Check sheet for the modelled part. Datum: model origin and axes. Units: mm. Face numbers are marked on the shaded views. A direction names the side the tool comes from. Round coordinates to 2 decimals unless told otherwise and drop trailing zeros. Write each loop counter-clockwise with the first axis right and the second up, starting at its lowest first coordinate (ties: lowest second). Pieces come first, ordered by that corner, then holes.
Item 1: Material ranges on line 1 along Z through (x, y) = (9.5, 5); line 2 along Y through (x, z) = (10, 6); line 3 along Z through (x, y) = (16.2, -19.05), recorded low to high.
Item 2: Section check A-A, the plane y = -0.5. Record the cut outline in (x, z), plus the area to 3 significant figures.
Item 3: Release check for a two-part mould opening along Z. For the marked faces 1, 2 and 3 record: pulls with the +Z half, pulls with the -Z half, needs draft (parallel to the pull), parting line crosses it, or undercut.
Item 4: Section check B-B, the plane x = 16.2. Record the cut outline in (y, z), plus the area to 3 significant figures.
Item 5: Set-up check for the marked faces 4 and 5: record each of +Z, -Z, +X, -X, +Y, -Y from which the full face is reachable in a straight line by a thin tool's end or side.
Item 6: Section check D-D, the plane y = -11. Record the cut outline in (x, z).
Item 7: Section check C-C, the plane x = 4. Record the cut outline in (y, z).
Item 8: Depth check by flat-ended pin: pin 1 (9 mm diameter, centred on x = 16, z = 0.5, fed in from +Y); pin 2 (4 mm diameter, centred on x = 11, z = 5, fed in from +Y). Enter the tip coordinate at first touch or a pass-through.
from build123d import *

# Parameters (mm, degrees)
TUBE_SQUARE_40_X_40_X_2_6_1_DEPTH = 35
CUT_EXTRUDE1_DEPTH                = 57.789083458
M12_CLEARANCE_HOLE1_D             = 13.5
M12_CLEARANCE_HOLE1_DEPTH         = 3.15
M12_CLEARANCE_HOLE1_TIP           = 4.055809178


with BuildPart() as part:
    # Sketch11 → Tube (square) 40 X 40 X 2.6(1) (new body)
    with BuildSketch(Plane.YZ):
        with BuildLine():
            Line((-14.8, -20), (14.8, -20))
            ThreePointArc((14.8, -20), (18.476955262, -18.476955262), (20, -14.8))
            Line((20, -14.8), (20, 14.8))
            ThreePointArc((20, 14.8), (18.476955262, 18.476955262), (14.8, 20))
            Line((14.8, 20), (-14.8, 20))
            ThreePointArc((-14.8, 20), (-18.476955262, 18.476955262), (-20, 14.8))
            Line((-20, 14.8), (-20, -14.8))
            ThreePointArc((-20, -14.8), (-18.476955262, -18.476955262), (-14.8, -20))
        make_face()
        with BuildLine():
            Line((-14.8, -17.4), (14.8, -17.4))
            ThreePointArc((14.8, -17.4), (16.638477631, -16.638477631), (17.4, -14.8))
            Line((17.4, -14.8), (17.4, 14.8))
            ThreePointArc((17.4, 14.8), (16.638477631, 16.638477631), (14.8, 17.4))
            Line((14.8, 17.4), (-14.8, 17.4))
            ThreePointArc((-14.8, 17.4), (-16.638477631, 16.638477631), (-17.4, 14.8))
            Line((-17.4, 14.8), (-17.4, -14.8))
            ThreePointArc((-17.4, -14.8), (-16.638477631, -16.638477631), (-14.8, -17.4))
        make_face(mode=Mode.SUBTRACT)
    extrude(amount=TUBE_SQUARE_40_X_40_X_2_6_1_DEPTH)

    # Sketch13 → Cut-Extrude1 (cut, through all)
    with BuildSketch(Plane.XY.offset(20)):
        Polygon((-5, 20), (35, -20), (35, 20), align=None)
    extrude(amount=-CUT_EXTRUDE1_DEPTH, mode=Mode.SUBTRACT)

    # M12 Clearance Hole1
    with Locations(Plane(origin=(0, -17.4, 0), x_dir=(1, 0, 0), z_dir=(0, 1, 0))):
        with Locations((16.2, 0)):
            Hole(M12_CLEARANCE_HOLE1_D / 2, depth=M12_CLEARANCE_HOLE1_DEPTH)
            with Locations((0, 0, -(M12_CLEARANCE_HOLE1_DEPTH + M12_CLEARANCE_HOLE1_TIP / 2))):  # 118° drill point
                Cone(0, M12_CLEARANCE_HOLE1_D / 2, M12_CLEARANCE_HOLE1_TIP, mode=Mode.SUBTRACT)


solid = part.part
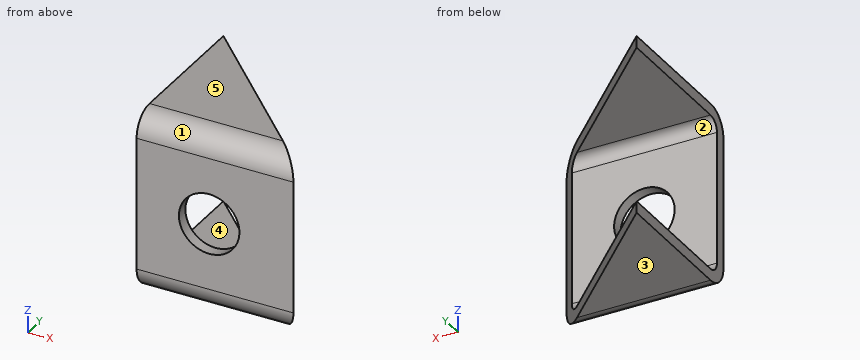
Values found:
1. line 1: z = -20 to -17.4, 17.4 to 20
1. line 2: y = -20 to -17.4
1. line 3: z = -17.8 to -6.75, 6.75 to 17.8
2. outline: (0, -20) - (15.5, -20) - (15.5, -17.4) - (0, -17.4) - close; (0, 17.4) - (15.5, 17.4) - (15.5, 20) - (0, 20) - close
2. area: 80.6 mm2
3. face 1: pulls with the +Z half
3. face 2: undercut
3. face 3: pulls with the -Z half
4. outline: (-20, -14.8) arc R5.2 ccw to (-14.8, -20) - (-1.2, -20) - (-1.2, -17.4) - (-14.8, -17.4) arc R2.6 cw to (-17.4, -14.8) - (-17.4, -6.75) - (-20, -6.75) - close; (-20, 6.75) - (-17.4, 6.75) - (-17.4, 14.8) arc R2.6 cw to (-14.8, 17.4) - (-1.2, 17.4) - (-1.2, 20) - (-14.8, 20) arc R5.2 ccw to (-20, 14.8) - close
4. area: 144 mm2
5. face 4: +X, -X, +Y
5. face 5: +Z, +X, -X, +Y, -Y
6. outline: (0, -20) - (26, -20) - (26, -17.4) - (0, -17.4) - close; (0, 17.4) - (26, 17.4) - (26, 20) - (0, 20) - close
7. outline: (-20, -14.8) arc R5.2 ccw to (-14.8, -20) - (11, -20) - (11, -17.4) - (-14.8, -17.4) arc R2.6 cw to (-17.4, -14.8) - (-17.4, 14.8) arc R2.6 cw to (-14.8, 17.4) - (11, 17.4) - (11, 20) - (-14.8, 20) arc R5.2 ccw to (-20, 14.8) - close
8. pin 1: passes through
8. pin 2: stops at y = -17.4
